For this review, take the finished solid that the model builds, in its own axes (mm). Face numbers are marked on the shaded views. A direction names the side the tool comes from. Coordinates: 2 decimals unless noted, no trailing zeros. Order: outer loops, then holes, each group sorted by start corner. A loop starts at its lowest first (then second) coordinate and runs counter-clockwise, first axis right, second up. Notation, with made-up numbers: (39.5, 59) -> (84.5, 59) arc R24 cw to (84.5, 91) -> close; hole circle Ø5 at (21, 80). An arc over 180 degrees is marked (long way). Answer as a JSON object with one key per item and string values. Group by question number.
1) Add section B-B, the plane y = 6.5. Write out the cut boundary in (x, z), then the cut area to 3 significant figures.
2) Draft analysis for pull direction Z (two halves, no side actions). For the marked faces 3, 4, 5 and 6, state which applies: +Z half, -Z half, draft (parallel to the pull), parting line (faces both ways), or undercut.
3) Add section C-C, the plane x = 4.75. Write out the cut boundary in (y, z), then the cut area to 3 significant figures.
4) Wall thickness on L1, parallel to X at y = 9, z = -6.25: over which ranges is the line inside the solid? List them lowest first.
5) Add section A-A, the plane z = -1.25. Write out the cut boundary in (x, y).
6) Machinability: for the marked faces 1 and 2, which of the approach directions +Z, -Z, +X, -X, +Y, -Y give a long, thin tool a straight path to every point of the face, cutting with its end or side? Answer none if there is none.
from build123d import *

# Parameters (mm, degrees)
SKETCH1_W           = 25
SKETCH1_H           = 25
SKETCH1_W_2         = 15
SKETCH1_H_2         = 15
BOSS_EXTRUDE1_DEPTH = 10
CUT_EXTRUDE1_DEPTH  = 0.5


with BuildPart() as part:
    # Sketch1 → Boss-Extrude1 (new body)
    with BuildSketch(Plane(origin=(0, 0, 0), x_dir=(1, 0, 0), z_dir=(0, 1, 0))):
        Rectangle(SKETCH1_W, SKETCH1_H)
        Rectangle(SKETCH1_W_2, SKETCH1_H_2, mode=Mode.SUBTRACT)
    extrude(amount=BOSS_EXTRUDE1_DEPTH)

    # Sketch2 → Cut-Extrude1 (cut)
    with BuildSketch(Plane(origin=(0, 10, 0), x_dir=(1, 0, 0), z_dir=(0, 1, 0))):
        Polygon((-3.273397436, -9.383333333), (-3.05418336, -9.383333333), (-2.5, -10.249165331), (-1.94581664, -9.383333333), (-1.726602564, -9.383333333), (-2.390180956, -10.420466079), (-1.699465812, -11.5), (-1.918679888, -11.5), (-2.5, -10.591766827), (-3.081320112, -11.5), (-3.300534188, -11.5), (-2.609395032, -10.420466079), align=None)
        Polygon((-11.364316239, 0.145833333), (-11.092418703, 0.145833333), (-10.39703943, -0.991048177), (-9.702720186, 0.145833333), (-9.43082265, 0.145833333), (-10.278846154, -1.24227514), (-10.278846154, -2.5), (-10.516292735, -2.5), (-10.516292735, -1.24227514), align=None)
    extrude(amount=-CUT_EXTRUDE1_DEPTH, mode=Mode.SUBTRACT)


solid = part.part
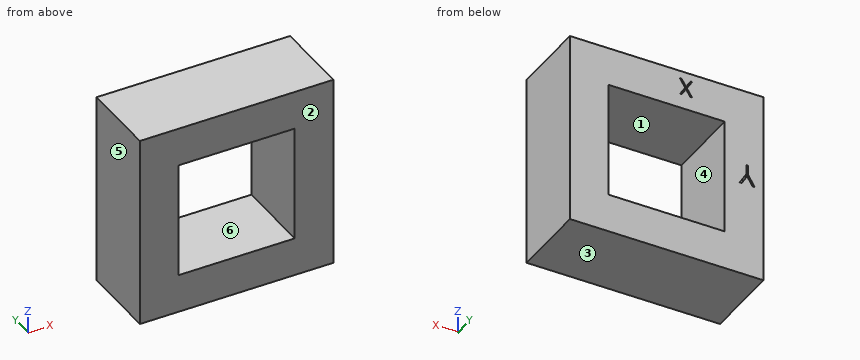
Output values:
{
 "1": {"outline": "(-12.5, -12.5) -> (12.5, -12.5) -> (12.5, 12.5) -> (-12.5, 12.5) -> close; hole (-7.5, -7.5) -> (7.5, -7.5) -> (7.5, 7.5) -> (-7.5, 7.5) -> close", "area": "400 mm²"},
 "2": {"face 3": "-Z half", "face 4": "undercut", "face 5": "draft", "face 6": "undercut"},
 "3": {"outline": "(0, -12.5) -> (10, -12.5) -> (10, -7.5) -> (0, -7.5) -> close; (0, 7.5) -> (10, 7.5) -> (10, 12.5) -> (0, 12.5) -> close", "area": "100 mm²"},
 "4": {"L1": "x = -12.5 to -7.5, 7.5 to 12.5"},
 "5": {"outline": "(-12.5, 0) -> (-7.5, 0) -> (-7.5, 10) -> (-12.5, 10) -> close; (7.5, 0) -> (12.5, 0) -> (12.5, 10) -> (7.5, 10) -> close"},
 "6": {"face 1": "+Y, -Y", "face 2": "+Z, -Z, +X, -X, -Y"}
}
